Geometry check sheet. Reference: the model listing, model coordinates, mm. A direction names the side the tool comes from. Coordinates: 2 decimals unless noted, no trailing zeros. Loops run counter-clockwise (first coordinate to the right, second up) from the corner with the lowest first, then second, coordinate; pieces in that order, holes last.
from build123d import *

# Parameters (mm, degrees)
BOSS_EXTRUDE1_DEPTH = 21
SKETCH3_W           = 24
SKETCH3_H           = 15
CUT_EXTRUDE1_DEPTH  = 59.037403457
FILLET1_R           = 1


with BuildPart() as part:
    # Sketch2 → Boss-Extrude1 (new, symmetric)
    with BuildSketch(Plane(origin=(0, 0, 0), x_dir=(0, 0, -1), z_dir=(1, 0, 0))):
        with BuildLine():
            Line((0, 0), (0, -6.35))
            Line((0, -6.35), (-3.81, -6.35))
            Line((-3.81, -6.35), (-3.81, 8.65))
            Line((-3.81, 8.65), (31.19, 8.65))
            Line((31.19, 8.65), (31.19, -35.56))
            Line((31.19, -35.56), (25.4, -35.56))
            ThreePointArc((25.4, -35.56), (23.276174446, -17.292737452), (17.018, 0))
            Line((17.018, 0), (0, 0))
        make_face()
    extrude(amount=BOSS_EXTRUDE1_DEPTH, both=True)

    # Sketch3 → Cut-Extrude1 (cut, through all)
    with BuildSketch(Plane(origin=(0, 8.65, 0), x_dir=(1, 0, 0), z_dir=(0, 1, 0))):
        with Locations((0, 18.5)):
            Rectangle(SKETCH3_W, SKETCH3_H)
    extrude(amount=-CUT_EXTRUDE1_DEPTH, mode=Mode.SUBTRACT)

    # Fillet1
    fillet1_edges = [part.edges().sort_by_distance(p)[0] for p in [
        (-12, 8.65, -18.5),
        (0, 8.65, -11),
        (12, 8.65, -18.5),
        (0, 8.65, -26),
    ]]
    fillet(fillet1_edges, radius=FILLET1_R)


solid = part.part
(1) Sectioned sample at A-A on z = -13.5. Record the cut outline in (x, y), and give its area (3 significant figures).
Findings:
outline: (-21, 0) - (-12, 0) - (-12, 7.65) arc R1 ccw to (-13, 8.65) - (-21, 8.65) - close; (12, 0) - (21, 0) - (21, 8.65) - (13, 8.65) arc R1 ccw to (12, 7.65) - close
area: 155 mm2
(2) Sectioned sample at B-B on x = 1. Record the cut outline in (y, z), and give its area (3 significant figures).
Findings:
outline: (-35.56, -31.19) - (8.65, -31.19) - (8.65, -27) arc R1 ccw to (7.65, -26) - (-35.56, -26) - close; (-6.35, 0) - (0, 0) - (0, -11) - (7.65, -11) arc R1 ccw to (8.65, -10) - (8.65, 3.81) - (-6.35, 3.81) - close
area: 381 mm2
(3) Gauge pin test, flat ends, axial feed: pin 1 Ø10 at (x, y) = (-15.5, -14.5) entering from +Z; pin 2 Ø1.1 at (x, z) = (0.5, 1.5) entering from -Y; pin 3 Ø12 at (y, z) = (-10, -7) entering from +X; pin 4 Ø12 at (x, y) = (5.5, -22) entering from +Z. Record the tip position at first contact, or that the pin passes through.
Findings:
pin 1: stops at z = -21.01
pin 2: stops at y = -6.35
pin 3: passes through
pin 4: stops at z = -26
(4) Draft check along X on faces 4 (the flat face through (-21, -3, -22)), 5 (the flat face through (0, 4, -11)), 6 (the flat face through (0, -35.56, -28)). Enter one of: +X half, -X half, draft (parallel to the pull), parting line (faces both ways), or undercut.
Findings:
face 4: -X half
face 5: undercut
face 6: draft
(5) Scan lines: L1, parallel to Z at x = 4, y = 7.5; L2, parallel to X at y = 7.5, z = -13; L3, parallel to Z at x = 16, y = -9.5. Record each from-to range of solid material in increasing order.
Findings:
L1: z = -31.19 to -26, -11 to 3.81
L2: x = -21 to -12, 12 to 21
L3: z = -31.19 to -21.01
(6) Access from +Z, -Z, +X, -X, +Y, -Y to the whole of each face (thin tool, end or side, straight path). Record for faces 1 (the flat face through (0, -6.35, 2)), 2 (the flat face through (0, -14, -26)), 3 (the flat face through (0, 0, -7)).
Findings:
face 1: +Z, +X, -X, -Y
face 2: +Y, -Y
face 3: +X, -X, -Y
(7) Sectioned sample at D-D on x = -16. Record the cut outline in (y, z).
Findings:
outline: (-35.56, -31.19) - (8.65, -31.19) - (8.65, 3.81) - (-6.35, 3.81) - (-6.35, 0) - (0, 0) - (0, -17.02) arc R79.62 cw to (-35.56, -25.4) - close
(8) Sectioned sample at C-C on y = -4.5. Record the cut outline in (x, z), and give its area (3 significant figures).
Findings:
outline: (-21, -31.19) - (21, -31.19) - (21, -19.09) - (12, -19.09) - (12, -26) - (-12, -26) - (-12, -19.09) - (-21, -19.09) - close; (-21, 0) - (21, 0) - (21, 3.81) - (-21, 3.81) - close
area: 502 mm2
